Solid Edge part; units mm, degrees
sketch "Sketch1" plane through (0, 0, 0) normal (0, 0, 1) x (1, 0, 0)
  line L0 (-20, -15) -> (100, -15)
  line L1 (100, -15) -> (100, 85)
  line L2 (100, 85) -> (-20, 85)
  line L3 (-20, 85) -> (-20, -15)
  dimension "D1" = 20
  dimension "D2" = 20
extrude "Protrusion1" add sketch "Sketch1" along normal blind 50
shell "Parede" thickness 5 removed faces 1 at (-1.2, 2.6667, 50)
sketch "Sketch2" plane through (100, 0, 50) normal (1, 0, 0) x (0, 0, -1)
  line L0 (45, 67.0982) -> (31, 67.0982)
  line L1 (31, 67.0982) -> (31, 57.5982)
  line L2 (31, 57.5982) -> (45, 57.5982)
  line L3 (45, 67.0982) -> (45, 57.5982)
  line L4 (45, 37.9671) -> (45, 25.9671)
  line L5 (35, 25.9671) -> (45, 25.9671)
  line L6 (35, 37.9671) -> (35, 25.9671)
  line L7 (45, 37.9671) -> (35, 37.9671)
extrude "Cutout1" cut sketch "Sketch2" against normal up to next
sketch "Sketch3" plane through (2.5, 0, 5) normal (0, 0, 1) x (1, 0, 0)
  line L0 (25.4753, 67.2334) -> (25.4753, 70)
  line L1 (25.4753, 70) -> (92.5, 70)
  line L2 (92.5, 70) -> (92.5, 72)
  line L3 (92.5, 72) -> (24.9753, 72)
  line L4 (23.4753, 70.5) -> (24.9753, 72)
  line L5 (23.4753, 70.5) -> (23.4753, 68.092)
  line L6 (21.1849, 65.9162) -> (23.4753, 68.092)
  line L7 (21.1849, 30.6261) -> (21.1849, 65.9162)
  line L8 (23.4753, 28.2151) -> (21.1849, 30.6261)
  line L9 (23.4753, 16.8218) -> (23.4753, 28.2151)
  line L10 (26.002, 13.874) -> (23.4753, 16.8218)
  line L11 (92.5, 13.874) -> (26.002, 13.874)
  line L12 (92.5, 15.874) -> (92.5, 13.874)
  line L13 (92.5, 15.874) -> (26.9219, 15.874)
  line L14 (26.9219, 15.874) -> (25.4753, 17.5616)
  line L15 (25.4753, 17.5616) -> (25.4753, 29.0137)
  line L16 (25.4753, 29.0137) -> (23.1849, 31.4246)
  line L17 (23.1849, 31.4246) -> (23.1849, 65.0575)
  line L18 (23.1849, 65.0575) -> (25.4753, 67.2334)
  circle A0 centre (25.4753, 62.4055) radius 1.3122
  circle A1 centre (25.4753, 34.1973) radius 1.3122
  circle A2 centre (76.8288, 18.8877) radius 1.3122
extrude "Parede_Arduino" add sketch "Sketch3" along normal blind 10
fillet "Round_1" radius 5 7 edges at (-20, -15, 25) (100, -15, 25) (100, 85, 25) (-20, 85, 25) (-15, -10, 27.5) (-15, 80, 27.5) (95, -10, 27.5)
The model under review builds one solid part; all positions refer to its coordinate system, in mm. A direction names the side the tool comes from. Round coordinates to 2 decimals unless told otherwise and drop trailing zeros. Loops run counter-clockwise (first coordinate to the right, second up) from the corner with the lowest first, then second, coordinate; pieces in that order, holes last. Notation, with made-up numbers: (34.25, 10) -> (81.25, 10) arc R17 cw to (81.25, 33) -> close; hole circle Ø8 at (1, -7). An arc over 180 degrees is marked (long way). Answer as a JSON object with one key per item and string values. Group by question number.
1) We need section C-C on y = 45.5. Write out the cut boundary in (x, z).
2) For faces 1 (the face through (25.975, 22, 10)), 2 (the face through (99, 83, 25)), list the 3-axis set-ups (+Z, -Z, +X, -X, +Y, -Y) from which the entire face can be reached by the end or side of a thin tool; tool diameter is ignored.
3) For line 1 (X direction, y = 43.5, z = 10); line 2 (Y direction, x = 55, z = 6.5); line 3 (X direction, y = 14.5, z = 34.5), list the stretches that pass through material, from the lowest coordinate up. Write a range as [from, to].
4) For pin 1 Ø16 at (x, y) = (63, 46) entering from +Z; pin 2 Ø4 at (x, z) = (97.5, 8.5) entering from -Y; pin 3 Ø0.8 at (x, y) = (28.5, 34) entering from +Z, all flat-tipped, find the tip position at first contact; note any pin that passes through.
5) We need section B-B on z = 33. Write out the cut boundary in (x, y).
6) We need section D-D on x = 17. Write out the cut boundary in (y, z).
7) Mouldability with a two-part tool opening along Z and no side actions: class faces 3 (the face through (98, 62, 19)), 4 (the face through (98, 32, 15)), 5 (the face through (39, -10, 27)), 6 (the face through (25, 43, 15)) as released by +Z, released by -Z, zero draft, split by the parting line, or undercut.
8) We need section A-A on x = 68. Write out the cut boundary in (y, z).
Result set:
{
 "1": {"outline": "(-20, 0) -> (100, 0) -> (100, 50) -> (95, 50) -> (95, 5) -> (25.68, 5) -> (25.68, 15) -> (23.68, 15) -> (23.68, 5) -> (-15, 5) -> (-15, 50) -> (-20, 50) -> close"},
 "2": {"face 1": "+Z", "face 2": "+Z, -Z, +X, +Y"},
 "3": {"line 1": "[-20, -15], [23.68, 25.68], [95, 100]", "line 2": "[-15, -10], [13.87, 15.87], [70, 72], [80, 85]", "line 3": "[-20, -15], [95, 100]"},
 "4": {"pin 1": "z = 5", "pin 2": "y = -14.97", "pin 3": "z = 15"},
 "5": {"outline": "(-20, -10) arc R5 ccw to (-15, -15) -> (95, -15) arc R5 ccw to (100, -10) -> (100, 80) arc R5 ccw to (95, 85) -> (-15, 85) arc R5 ccw to (-20, 80) -> close; hole (-15, -5) arc R5 ccw to (-10, -10) -> (90, -10) arc R5 ccw to (95, -5) -> (95, 80) -> (-10, 80) arc R5 ccw to (-15, 75) -> close"},
 "6": {"outline": "(-15, 0) -> (85, 0) -> (85, 50) -> (80, 50) -> (80, 5) -> (-10, 5) -> (-10, 50) -> (-15, 50) -> close"},
 "7": {"face 3": "undercut", "face 4": "undercut", "face 5": "zero draft", "face 6": "released by +Z"},
 "8": {"outline": "(-15, 0) -> (85, 0) -> (85, 50) -> (80, 50) -> (80, 5) -> (72, 5) -> (72, 15) -> (70, 15) -> (70, 5) -> (15.87, 5) -> (15.87, 15) -> (13.87, 15) -> (13.87, 5) -> (-10, 5) -> (-10, 50) -> (-15, 50) -> close"}
}
